Autodesk Inventor part; units mm, degrees
ref_plane "YZ Plane" through (0, 0, 0) normal (1, 0, 0) x (0, 1, 0)
ref_plane "XZ Plane" through (0, 0, 0) normal (0, 1, 0) x (-1, 0, 0)
ref_plane "XY Plane" through (0, 0, 0) normal (0, 0, 1) x (1, 0, 0)
sketch "Skizze1" plane through (0, 0, 0) normal (0, 0, 1) x (1, 0, 0)
  line L0 (0, 12) -> (62, 12)
  line L1 (62, -12) -> (0, -12)
  line L2 (0, -12) -> (0, 12)
  line L3 (-14.2, 0) -> (85.2, 0)
  line L4 (62, -7) -> (71, -7)
  line L5 (71, -7) -> (71, 7)
  line L6 (71, 7) -> (62, 7)
  line L7 (62, 12) -> (62, 7)
  line L8 (62, -7) -> (62, -12)
  point P0 (0, 0)
  dimension "d0" = 24
  dimension "d1" = 62
  dimension "d29" = 14
  dimension "d30" = 9
extrude "Extrusion1" add sketch "Skizze1" along normal blind 4
sketch "Skizze5" plane through (0, 0, 0) normal (0, 0, -1) x (-1, 0, 0)
  line L0 (0, -12) -> (0, 12) construction
  line L1 (-85.2, 0) -> (14.2, 0) construction
  line L2 (0, 12) -> (0, -12)
  line L3 (0, -8) -> (-6, -8)
  line L4 (-8, -6) -> (-8, 6)
  line L5 (-6, 8) -> (0, 8)
  line L6 (0, 8) -> (0, -8)
  arc A0 (-8, -6) -> (-6, -8) centre (-6, -6) ccw
  arc A1 (-6, 8) -> (-8, 6) centre (-6, 6) ccw
  point P0 (0, 0)
  dimension "d37" = 2
  dimension "d38" = 4
  dimension "d39" = 8
extrude "Extrusion3" cut sketch "Skizze5" against normal blind 2
sketch "Skizze6" plane through (0, 0, 4) normal (0, 0, 1) x (1, 0, 0)
  line L0 (0, 12) -> (0, -12) construction
  line L1 (-24.0571, 0) -> (86.8428, 0) construction
  line L2 (0, 7.9) -> (-5.8, 7.9)
  line L3 (-7.8, 5.9) -> (-7.8, -5.9)
  line L4 (-5.8, -7.9) -> (0, -7.9)
  line L5 (0, -7.9) -> (0, 7.9)
  arc A0 (-5.8, 7.9) -> (-7.8, 5.9) centre (-5.8, 5.9) ccw
  arc A1 (-7.8, -5.9) -> (-5.8, -7.9) centre (-5.8, -5.9) ccw
  point P0 (0, 0)
  dimension "d42" = 2
  dimension "d43" = 4.1
  dimension "d44" = 7.8
extrude "Extrusion4" add sketch "Skizze6" against normal blind 2
sketch "Skizze2" plane through (0, 0, 4) normal (0, 0, 1) x (1, 0, 0)
  line L0 (62, 12) -> (0, 12)
  line L1 (0, 12) -> (0, -12)
  line L2 (0, 12) -> (4, 12)
  line L3 (4, 12) -> (4, -12)
  line L4 (4, -12) -> (0, -12)
  line L5 (0, -12) -> (0, 12)
  point P0 (0, 0)
  dimension "d4" = 4
extrude "Extrusion2" [suppressed]
sketch "Skizze3" plane through (0, 0, 2) normal (0, 0, 1) x (1, 0, 0)
  line L0 (0, 16.8) -> (0, -16.8)
  line L1 (-15, 0) -> (90, 0)
  point P0 (0, 0)
  point P1 (2, 0)
  dimension "d7" = 2
hole "Bohrung1" [suppressed]
pattern_linear "Rechteckige Anordnung1" [suppressed]
sketch "Skizze4" plane through (0, 0, 4) normal (0, 0, 1) x (1, 0, 0)
  line L0 (-14.2, 0) -> (85.2, 0)
  line L1 (62, -12) -> (62, 12)
  line L2 (71, -7) -> (71, 7) construction
  point P0 (0, 0)
  point P1 (62, 4)
  point P2 (62, -4)
  dimension "d31" = 8
  dimension "d36" = 0
hole "Bohrung2" at (62, -4, 4) at (62, 4, 4) direction (0, 0, -1) diameter 3.242 end through all
fillet "Rundung1" radius 4 2 edges at (62, -7, 2) (62, 7, 2)
fillet "Rundung2" radius 1 4 edges at (62, -12, 2) (62, 12, 2) (71, -7, 2) (71, 7, 2)
sketch "Skizze7" plane through (0, 0, 0) normal (0, 0, 1) x (1, 0, 0)
  line L0 (-4, -4) -> (4, -4) construction
  line L1 (4, -4) -> (4, 4) construction
  line L2 (4, 4) -> (-4, 4) construction
  line L3 (-4, 4) -> (-4, -4) construction
  line L4 (0, 5.6) -> (0, -5.6) construction
  line L5 (-5.6, 0) -> (5.6, 0) construction
  point P0 (0, 0)
  dimension "d48" = 8
  dimension "d49" = 8
hole "Bohrung3" at (4, -4, 0) at (4, 4, 0) at (-4, 4, 0) at (-4, -4, 0) direction (0, 0, 1) diameter 2.459 end through all
fillet "Rundung3" radius 2 4 edges at (0, -8, 1) (0, 8, 1) (0, 7.9, 3) (0, -7.9, 3)
properties part number "Kicker Eisen" material "Stahl, unlegiert"
For this review, take the finished solid that the model builds, in its own axes (mm). A direction names the side the tool comes from. Round coordinates to 2 decimals unless told otherwise and drop trailing zeros. Order: outer loops, then holes, each group sorted by start corner. A loop starts at its lowest first (then second) coordinate and runs counter-clockwise, first axis right, second up. Notation, with made-up numbers: (-5.5, -25) -> (27.5, -25) arc R24 cw to (27.5, 4) -> close; hole circle Ø4 at (15.5, 33.5). An arc over 180 degrees is marked (long way). Put each result on its own line as item: value.
Q1. Mouldability with a two-part tool opening along Y and no side actions: class faces 1 (the cylindrical face through (0.6, -8.57, 1.01)), 2 (the flat face through (31, -12, 2)), 3 (the cylindrical face through (-7.2, 7.33, 3.01)), 4 (the cylindrical face through (63.582, 4.351, 1.972)) as pulls with the +Y half, pulls with the -Y half, needs draft (parallel to the pull), parting line crosses it, or undercut.
Check result:
face 1: undercut
face 2: pulls with the -Y half
face 3: pulls with the +Y half
face 4: undercut
Q2. Add section C-C on z = 2.65. State how many separate pieces and enclosed holes the cut face has, plus the area to 3 significant figures.
Check result:
separate pieces: 1
enclosed holes: 6
area: 1,710 mm2
Q3. Machinability: for faces 5 (the flat face through (0, -11, 2)), 6 (the flat face through (68, -7, 2)), 7 (the flat face through (4, -8, 1)), 8 (the flat face through (68, 7, 2)), which of the approach directions +Z, -Z, +X, -X, +Y, -Y give a long, thin tool a straight path to every point of the face, cutting with its end or side? Answer none if there is none.
Check result:
face 5: +Z, -Z, -X, -Y
face 6: +Z, -Z, +X, -Y
face 7: -Z, -X
face 8: +Z, -Z, +X, +Y
Q4. Insertion check: pin 1 Ø1 at (x, z) = (-4.5, 2.5) entering from -Y; pin 2 Ø0.6 at (y, z) = (-1, 0.5) entering from -X; pin 3 Ø2 at (x, z) = (-3.5, 3) entering from +Y. Each pin has a flat end and moves straight along its axis. Give the tip position at first contact, or say it passes through.
Check result:
pin 1: y = -7.9
pin 2: x = 8
pin 3: y = 7.9
Q5. For probe 1 along Y at (x, z) = (4, 3.1); probe 2 along Y at (x, z) = (-4, 2.85); probe 3 along X at (y, z) = (4, 3.05), list the stretches that pass through material, from the lowest coordinate up. Write a range as [from, to].
Check result:
probe 1: [-12, -5.23], [-2.77, 2.77], [5.23, 12]
probe 2: [-7.9, -5.23], [-2.77, 2.77], [5.23, 7.9]
probe 3: [-7.8, -5.23], [-2.77, 2.77], [5.23, 60.38], [63.62, 71]
Q6. Add section B-B on x = -4. Write out the cut boundary in (y, z).
Check result:
outline: (-7.9, 2) -> (-5.23, 2) -> (-5.23, 4) -> (-7.9, 4) -> close; (-2.77, 2) -> (2.77, 2) -> (2.77, 4) -> (-2.77, 4) -> close; (5.23, 2) -> (7.9, 2) -> (7.9, 4) -> (5.23, 4) -> close
Q7. Add section D-D on y = -4.25. Write out the cut boundary in (x, z), plus the area to 3 significant figures.
Check result:
outline: (-7.8, 2) -> (-5.2, 2) -> (-5.2, 4) -> (-7.8, 4) -> close; (-2.8, 2) -> (2.8, 2) -> (2.8, 4) -> (-2.8, 4) -> close; (5.2, 2) -> (8, 2) -> (8, 0) -> (60.4, 0) -> (60.4, 4) -> (5.2, 4) -> close; (63.6, 0) -> (71, 0) -> (71, 4) -> (63.6, 4) -> close
area: 261 mm2
Q8. Add section A-A on y = 4. Write out the cut boundary in (x, z).
Check result:
outline: (-7.8, 2) -> (-5.23, 2) -> (-5.23, 4) -> (-7.8, 4) -> close; (-2.77, 2) -> (2.77, 2) -> (2.77, 4) -> (-2.77, 4) -> close; (5.23, 2) -> (8, 2) -> (8, 0) -> (60.38, 0) -> (60.38, 4) -> (5.23, 4) -> close; (63.62, 0) -> (71, 0) -> (71, 4) -> (63.62, 4) -> close
